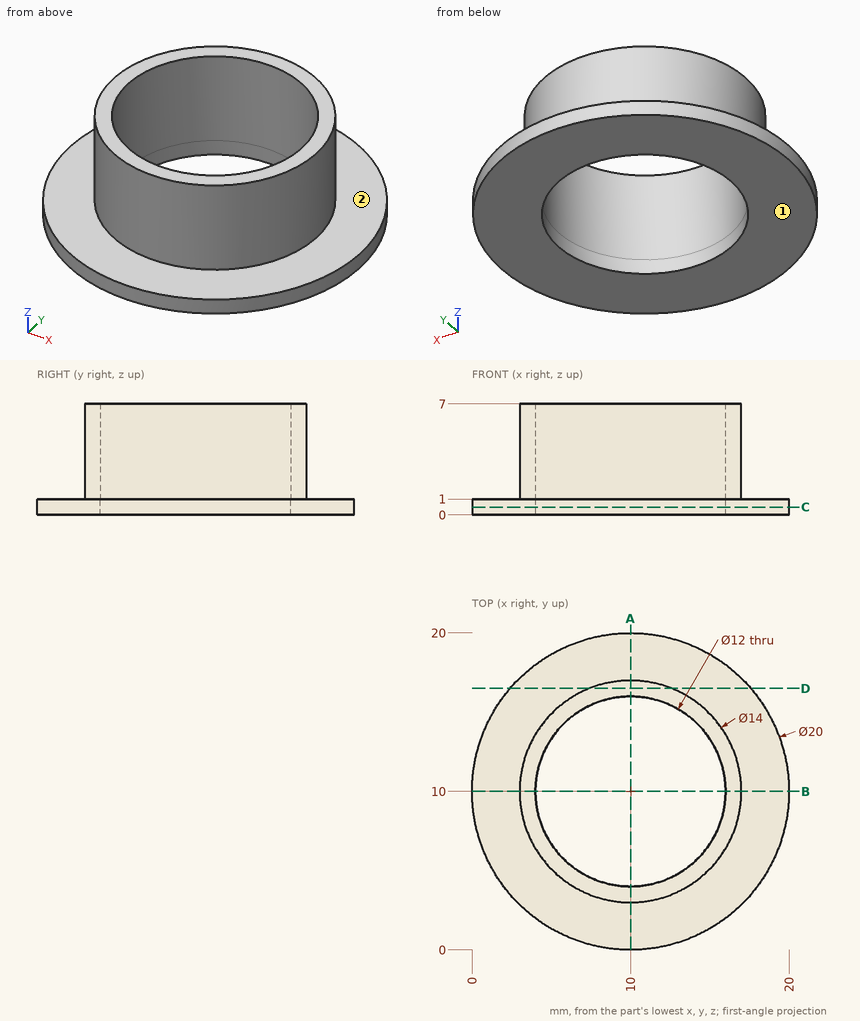
Check sheet for the drawn part. Datum: minimum x, y, z corner. Units: mm. A direction names the side the tool comes from. Round coordinates to 2 decimals unless told otherwise and drop trailing zeros. Order: outer loops, then holes, each group sorted by start corner. A loop starts at its lowest first (then second) coordinate and runs counter-clockwise, first axis right, second up. Notation, with made-up numbers: (27.25, 61.5) - (70.25, 61.5) arc R26 ccw to (70.25, 78.5) - close; hole circle Ø10 at (28.5, 68.5). An arc over 180 degrees is marked (long way). Use a Markdown table: item, result. Add a question column.
(1) Sectioned sample at C-C, the plane z = 0.5. Enter the section's corners in (x, y).
(2) Sectioned sample at D-D, the plane y = 16.5. Enter the section's corners in (x, z), and give its area (3 significant figures).
(3) Tool access check on the marked faces 1 and 2. Record the directions out of +Z, -Z, +X, -X, +Y, -Y that give a thin tool (end or side, any length) a straight path to the whole face; none if there is none.
(4) Depth check by flat-ended pin: pin 1 (1 mm diameter, centred on x = 16.5, z = 2, fed in from -Y); pin 2 (1.5 mm diameter, centred on x = 11, z = 1, fed in from +Y); pin 3 (11 mm diameter, centred on x = 10, y = 10, fed in from -Z); pin 4 (1 mm diameter, centred on y = 8.5, z = 2, fed in from +X). Enter the tip coordinate at first touch or a pass-through.
(5) Material ranges on line 1 along Y through (x, z) = (10, 5.65); line 2 along Y through (x, z) = (10, 0.55); line 3 along Z through (x, y) = (15.75, 17.5), recorded low to high. Write a range as [from, to].
(6) Sectioned sample at A-A, the plane x = 10. Enter the section's corners in (y, z), and give its area (3 significant figures).
Answers below:
| question | item | result |
|---|---|---|
| 1 | outline | circle Ø20 at (10, 10); hole circle Ø12 at (10, 10) |
| 2 | outline | (2.4, 0) - (17.6, 0) - (17.6, 1) - (12.6, 1) - (12.6, 7) - (7.4, 7) - (7.4, 1) - (2.4, 1) - close |
| 2 | area | 46.4 mm² |
| 3 | face 1 | -Z, +X, -X, +Y, -Y |
| 3 | face 2 | +Z |
| 4 | pin 1 | y = 6.39 |
| 4 | pin 2 | y = 20 |
| 4 | pin 3 | through |
| 4 | pin 4 | x = 16.93 |
| 5 | line 1 | [3, 4], [16, 17] |
| 5 | line 2 | [0, 4], [16, 20] |
| 5 | line 3 | [0, 1] |
| 6 | outline | (0, 0) - (4, 0) - (4, 7) - (3, 7) - (3, 1) - (0, 1) - close; (16, 0) - (20, 0) - (20, 1) - (17, 1) - (17, 7) - (16, 7) - close |
| 6 | area | 20.0 mm² |
